Design review of the part built by this model. Coordinates are the model's own, in mm. A direction names the side the tool comes from. Round coordinates to 2 decimals unless told otherwise and drop trailing zeros. Loops run counter-clockwise (first coordinate to the right, second up) from the corner with the lowest first, then second, coordinate; pieces in that order, holes last. Notation, with made-up numbers: (50, 89.5) - (84, 89.5) arc R8 cw to (84, 99.5) - close; hole circle Ø5 at (-12.75, 28). An arc over 180 degrees is marked (long way). Use one line per item in the form item = value. Start each with the question number.
(1) Machinability: for faces 1 (the flat face through (100.494, -18, -7)), 2 (the flat face through (3, 0, -8)), 3 (the flat face through (3, 2.5, -8)), which of the approach directions +Z, -Z, +X, -X, +Y, -Y give a long, thin tool a straight path to every point of the face, cutting with its end or side? Answer none if there is none.
(2) We need section A-A, the plane y = -12.5. Write out the cut boundary in (x, z), then the cut area to 3 significant figures.
(3) For pin 1 (3 mm diameter, centred on y = 1.5, z = -13.5, fed in from -X); pin 2 (2 mm diameter, centred on x = 56.5, z = 8.5, fed in from +Y); pin 3 (6 mm diameter, centred on y = -19, z = 14, fed in from -X), all flat-tipped, find the tip position at first contact; note any pin that passes through.
(4) We need section B-B, the plane z = -14. Write out the cut boundary in (x, y).
(5) We need section C-C, the plane z = 7. Write out the cut boundary in (x, y), then the cut area to 3 significant figures.
(6) Wall thickness on probe 1 along X at (y, z) = (-28, -28.5); probe 2 along Y at (x, z) = (72, -1); probe 3 along Z at (x, y) = (73, 1): over which ranges is each line inside the solid? List them lowest first. Write a range as [from, to].
from build123d import *

# Parameters (mm, degrees)
SKETCH_1_W          = 185
SKETCH_1_H          = 73
EXTRUDE_1_DEPTH     = 2.5
SKETCH_2_W          = 15
SKETCH_2_H          = 2.5
EXTRUDE_2_DEPTH     = 2.5
FILLET_2_R          = 1.25
SKETCH_3_W          = 73
SKETCH_3_H          = 38.5
EXTRUDE_3_DEPTH     = 2.5
FILLET_3_R          = 1.25
SKETCH_4_W          = 19
SKETCH_4_H          = 15
CUT_EXTRUDE_1_DEPTH = 2.5
SKETCH_5_W          = 4
SKETCH_5_H          = 4
CUT_EXTRUDE_2_DEPTH = 2.5


with BuildPart() as part:
    # 草图1 → 凸台-拉伸1 (new body)
    with BuildSketch(Plane(origin=(0, 0, 0), x_dir=(1, 0, 0), z_dir=(0, 1, 0))):
        with Locations((5.493520518, 7.607451404)):
            Rectangle(SKETCH_1_W, SKETCH_1_H)
    extrude(amount=EXTRUDE_1_DEPTH)

    # 草图2 → 凸台-拉伸2 (add)
    with BuildSketch(Plane.ZY.offset(87.006479482)):
        with Locations((-26.607451404, 1.25)):
            Rectangle(SKETCH_2_W, SKETCH_2_H)
        with Locations((11.392548596, 1.25)):
            Rectangle(SKETCH_2_W, SKETCH_2_H)
    extrude(amount=EXTRUDE_2_DEPTH)

    # 圆角2
    fillet_2_edges = [part.edges().sort_by_distance(p)[0] for p in [
        (-88.256479482, 2.5, 3.892548596),
        (-88.256479482, 0, 3.892548596),
        (-88.256479482, 0, 18.892548596),
        (-88.256479482, 2.5, 18.892548596),
        (-88.256479482, 0, -34.107451404),
        (-88.256479482, 2.5, -19.107451404),
        (-88.256479482, 0, -19.107451404),
        (-88.256479482, 2.5, -34.107451404),
    ]]
    fillet(fillet_2_edges, radius=FILLET_2_R - 0.0001)  # a hair under: the kernel refuses the full size

    # 草图3 → 凸台-拉伸3 (add)
    with BuildSketch(Plane(origin=(97.993520518, 0, 0), x_dir=(0, 0, -1), z_dir=(1, 0, 0))):
        with Locations((7.607451404, -14.25)):
            Rectangle(SKETCH_3_W, SKETCH_3_H)
    extrude(amount=EXTRUDE_3_DEPTH)

    # 圆角3
    fillet_3_edges = [part.edges().sort_by_distance(p)[0] for p in [
        (5.493520518, 0, -44.107451404),
        (5.493520518, 2.5, -44.107451404),
        (5.493520518, 0, 28.892548596),
        (5.493520518, 2.5, 28.892548596),
    ]]
    fillet(fillet_3_edges, radius=FILLET_3_R - 0.0001)  # a hair under: the kernel refuses the full size

    # 草图4 → 切除-拉伸1 (cut)
    with BuildSketch(Plane(origin=(100.493520518, 0, 0), x_dir=(0, 0, -1), z_dir=(1, 0, 0))):
        with Locations((14.607451404, -8)):
            Rectangle(SKETCH_4_W, SKETCH_4_H)
    extrude(amount=-CUT_EXTRUDE_1_DEPTH, mode=Mode.SUBTRACT)

    # 草图5 → 切除-拉伸2 (cut)
    with BuildSketch(Plane(origin=(0, 2.5, 0), x_dir=(1, 0, 0), z_dir=(0, 1, 0))):
        with Locations((26.493520518, 24.607451404)):
            Rectangle(SKETCH_5_W, SKETCH_5_H)
    extrude(amount=-CUT_EXTRUDE_2_DEPTH, mode=Mode.SUBTRACT)


solid = part.part
Data:
q1.face_1 = +Z, -Z, +X, +Y, -Y
q1.face_2 = +Z, -Z, -X, -Y
q1.face_3 = +Z, -Z, -X, +Y
q2.outline = (97.99, -44.11) - (100.49, -44.11) - (100.49, -24.11) - (97.99, -24.11) - close; (97.99, -5.11) - (100.49, -5.11) - (100.49, 28.89) - (97.99, 28.89) - close
q2.area = 135 mm^2
q3.pin_1 = -87.01
q3.pin_2 = 2.5
q3.pin_3 = 97.99
q4.outline = (-87.01, 0) - (97.99, 0) - (97.99, -0.5) - (100.49, -0.5) - (100.49, 5) - (97.99, 5) - (97.99, 2.5) - (-87.01, 2.5) - close; (97.99, -33.5) - (100.49, -33.5) - (100.49, -15.5) - (97.99, -15.5) - close
q5.outline = (-89.51, 0) - (97.99, 0) - (97.99, -33.5) - (100.49, -33.5) - (100.49, 5) - (97.99, 5) - (97.99, 2.5) - (-89.51, 2.5) - close
q5.area = 565 mm^2
q6.probe_1 = [97.99, 100.49]
q6.probe_2 = [0, 2.5]
q6.probe_3 = [-44.08, 28.87]
